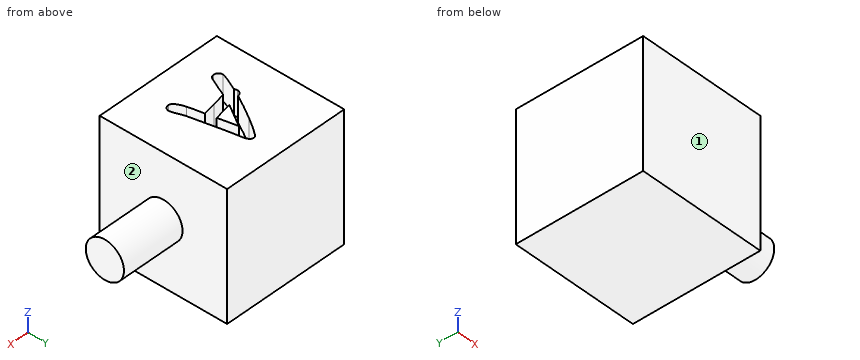
Autodesk Inventor part; units mm, degrees
ref_plane "YZ Plane" through (0, 0, 0) normal (1, 0, 0) x (0, 1, 0)
ref_plane "XZ Plane" through (0, 0, 0) normal (0, 1, 0) x (-1, 0, 0)
ref_plane "XY Plane" through (0, 0, 0) normal (0, 0, 1) x (1, 0, 0)
sketch "Sketch1" plane through (0, 0, 0) normal (1, 0, 0) x (0, 1, 0)
  line L0 (0, 0) -> (10, 0)
  line L1 (10, 0) -> (10, -10)
  line L2 (10, -10) -> (0, -10)
  line L3 (0, -10) -> (0, 0)
  dimension "d0" = 10
  dimension "d1" = 10
extrude "Extrusion1" add sketch "Sketch1" along normal blind 10
sketch "Sketch2" plane through (10, 0, 0) normal (1, 0, 0) x (0, 0, -1)
  circle A0 centre (5, 5) radius 1.5
  point P0 (0, 0)
  dimension "d4" = 3
extrude "Extrusion2" add sketch "Sketch2" along normal blind 5
sketch "Sketch4" plane through (0, 0, 0) normal (0, 0, 1) x (1, 0, 0)
  line L0 (1.8731, 7.9408) -> (4.4271, 7.9408) construction
  line L1 (4.4271, 7.9408) -> (4.4271, 4.8928) construction
  line L2 (4.4271, 4.8928) -> (1.8731, 4.8928) construction
  line L3 (1.8731, 4.8928) -> (1.8731, 7.9408) construction
  spline S0 degree 2 poles (6.5901, 2.2509) (6.243, 2.2509) (5.9854, 3.1396) knots 0 0 0 1 1 1
  spline S1 degree 2 poles (5.9854, 3.1396) (5.8854, 3.4814) (5.7382, 4.3281) knots 0 0 0 1 1 1
  spline S2 degree 2 poles (5.7382, 4.3281) (5.3543, 4.2755) (4.7338, 4.1388) knots 0 0 0 1 1 1
  line L4 (4.7338, 4.1388) -> (3.7347, 3.9337)
  spline S3 degree 2 poles (3.7347, 3.9337) (3.5454, 3.4394) (3.0826, 2.4876) knots 0 0 0 1 1 1
  spline S4 degree 2 poles (3.0826, 2.4876) (2.9617, 2.2772) (2.7566, 2.2772) knots 0 0 0 1 1 1
  spline S5 degree 2 poles (2.7566, 2.2772) (2.6041, 2.2772) (2.3674, 2.4981) (2.3674, 2.6558) knots 0 0 0 1 2 2 2
  spline S6 degree 2 poles (2.3674, 2.6558) (2.3674, 2.8399) (2.9354, 4.0336) knots 0 0 0 1 1 1
  spline S7 degree 2 poles (2.9354, 4.0336) (2.8723, 4.1335) (2.8723, 4.2597) knots 0 0 0 1 1 1
  spline S8 degree 2 poles (2.8723, 4.2597) (2.8723, 4.5647) (3.2404, 4.6541) knots 0 0 0 1 1 1
  spline S9 degree 2 poles (3.2404, 4.6541) (3.6716, 5.4587) (4.3289, 6.5104) knots 0 0 0 1 1 1
  spline S10 degree 2 poles (4.3289, 6.5104) (5.2229, 7.9408) (5.4437, 7.9408) knots 0 0 0 1 1 1
  spline S11 degree 2 poles (5.4437, 7.9408) (5.7382, 7.9408) (5.8486, 7.5253) knots 0 0 0 1 1 1
  line L5 (5.8486, 7.5253) -> (6.0853, 6.258)
  line L6 (6.0853, 6.258) -> (6.6479, 3.6339)
  line L7 (6.6479, 3.6339) -> (6.8636, 3.0397)
  spline S12 degree 2 poles (6.8636, 3.0397) (6.974, 2.7347) (6.974, 2.6296) knots 0 0 0 1 1 1
  spline S13 degree 2 poles (6.974, 2.6296) (6.974, 2.4718) (6.7426, 2.2509) (6.5901, 2.2509) knots 0 0 0 1 2 2 2
  line L8 (5.2597, 6.563) -> (4.1817, 4.8224)
  spline S14 degree 2 poles (4.1817, 4.8224) (4.6392, 4.9381) (5.5647, 5.1064) knots 0 0 0 1 1 1
  line L9 (5.5647, 5.1064) -> (5.2597, 6.563)
  point P0 (0, 0)
extrude "Extrusion4" cut sketch "Sketch4" against normal blind 2
properties part number "Adenosine"
Can you work these out from the model? Positions are in its coordinate system, mm. Face numbers are marked on the shaded views. A direction names the side the tool comes from. Coordinates: 2 decimals unless noted, no trailing zeros. Loops run counter-clockwise (first coordinate to the right, second up) from the corner with the lowest first, then second, coordinate; pieces in that order, holes last.
Item 1: Suppose I cut it at D-D (z = -4). Please give me the cut outline in (x, y), then the cut area to 3 significant figures.
Answers below:
outline: (0, 0) - (10, 0) - (10, 3.88) - (15, 3.88) - (15, 6.12) - (10, 6.12) - (10, 10) - (0, 10) - close
area: 111 mm2
Item 2: Please list where these lines run through material, in increasing order: L1, parallel to X at y = 2.5, z = -9; L2, parallel to Z at x = 2.5, y = 2.75; L3, parallel to Z at x = 14, y = 4.
Answers below:
L1: x = 0 to 10
L2: z = -10 to -2
L3: z = -6.12 to -3.88
Item 3: Suppose I cut it at C-C (y = 2). Please give me the cut outline in (x, z).
Answers below:
outline: (0, -10) - (10, -10) - (10, 0) - (0, 0) - close
Item 4: Suppose I cut it at B-B (x = 13.5). Please give me the cut outline in (y, z).
Answers below:
outline: circle Ø3 at (5, -5)
Item 5: Which directions (+Z, -Z, +X, -X, +Y, -Y) give clear straight access to the entire face, cutting with the end or side of a thin tool? Please do the marked faces 1 and 2.
Answers below:
face 1: +Z, -Z, +X, -X, -Y
face 2: +X
Item 6: Suppose I cut it at A-A (z = -5.25). Please give me the cut outline in (x, y).
Answers below:
outline: (0, 0) - (10, 0) - (10, 3.52) - (15, 3.52) - (15, 6.48) - (10, 6.48) - (10, 10) - (0, 10) - close
Item 7: I'm going to push a flat-ended pin straight in: pin 1 (1 mm diameter, centred on y = 4.5, z = -8, fed in from +X). Where does the tip first touch, or does it pass through?
Answers below:
pin 1: stops at x = 10
